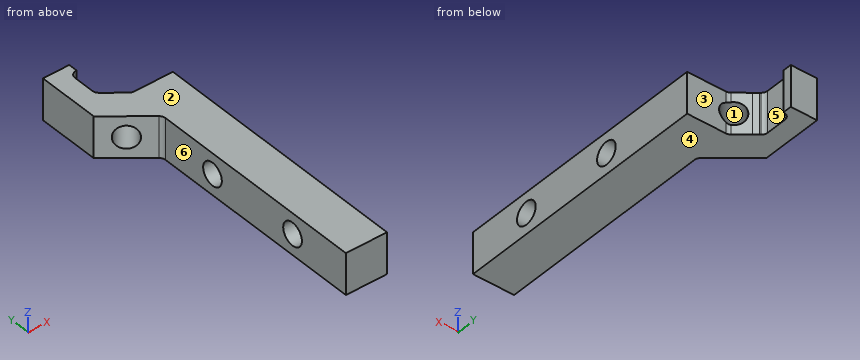
from build123d import *

# Parameters (mm, degrees)
BOSS_EXTRUDE1_DEPTH     = 12.7
CUT_EXTRUDE1_DEPTH      = 100.645019946
CUT_EXTRUDE1_DEPTH_BACK = 100.645019946
SKETCH6_R               = 3.5
SKETCH8_R               = 3.5
CUT_EXTRUDE2_DEPTH      = 315.511656717


with BuildPart() as part:
    # Sketch1 → Boss-Extrude1 (new body)
    with BuildSketch(Plane.XY):
        with BuildLine():
            Line((-312.7, 0), (-300, 0))
            Line((-300, 0), (-300, 80.249402298))
            Line((-300, 80.249402298), (-311.985474591, 80.249402298))
            ThreePointArc((-311.985474591, 80.249402298), (-312.658347569, 80.365989981), (-313.252771846, 80.702160342))
            Line((-313.252771846, 80.702160342), (-317.170141731, 83.91075489))
            Line((-317.170141731, 83.91075489), (-318.5, 85))
            Line((-318.5, 85), (-318.767297255, 85.21893478))
            ThreePointArc((-318.767297255, 85.21893478), (-319.307566667, 85.91019616), (-319.5, 86.766176735))
            Line((-319.5, 86.766176735), (-319.5, 93.25))
            ThreePointArc((-319.5, 93.25), (-318.914213562, 94.664213562), (-317.5, 95.25))
            Line((-317.5, 95.25), (-317.388555411, 95.25))
            Line((-317.388555411, 95.25), (-317.388555411, 96.25))
            Line((-317.388555411, 96.25), (-317.388555411, 98))
            Line((-317.388555411, 98), (-318.5, 98))
            Line((-318.5, 98), (-325.5, 98))
            Line((-325.5, 98), (-325.5, 85))
            Line((-325.5, 85), (-325.5, 82))
            Line((-325.5, 82), (-325.5, 79))
            Line((-325.5, 79), (-313.432702745, 69.116056102))
            ThreePointArc((-313.432702745, 69.116056102), (-312.892433333, 68.424794722), (-312.7, 67.568814146))
            Line((-312.7, 67.568814146), (-312.7, 63.3))
            Line((-312.7, 63.3), (-312.7, 60.3))
            Line((-312.7, 60.3), (-312.7, 0))
        make_face()
    extrude(amount=BOSS_EXTRUDE1_DEPTH)

    # Sketch6 → Cut-Extrude1 (cut, two sides: drawn at the far end of the back side and taken through both)
    with BuildSketch(Plane.ZY.offset(312.7).offset(-CUT_EXTRUDE1_DEPTH_BACK)):
        with Locations((6.35, 50)):
            Circle(SKETCH6_R)
        with Locations((6.35, 20)):
            Circle(SKETCH6_R)
    extrude(amount=CUT_EXTRUDE1_DEPTH + CUT_EXTRUDE1_DEPTH_BACK, mode=Mode.SUBTRACT)

    # Sketch8 → Cut-Extrude2 (cut, through all)
    with BuildSketch(Plane(origin=(-91.96558898, -112.280695929, 0), x_dir=(0.7736209776319443, -0.6336486273699289, 0), z_dir=(-0.6336486273699289, -0.7736209776319443, 0))):
        with Locations((-294.07263889, 6.35)):
            Circle(SKETCH8_R)
    extrude(amount=-CUT_EXTRUDE2_DEPTH, mode=Mode.SUBTRACT)


solid = part.part
Work out the finished part from the listing and answer in its coordinate system (mm). Face numbers are marked on the shaded views. A direction names the side the tool comes from. Give positions to 0.01 mm unless a question says otherwise; leave off trailing zeros. Write each loop counter-clockwise with the first axis right and the second up, starting at its lowest first coordinate (ties: lowest second). Pieces come first, ordered by that corner, then holes.
Q1. For a pull along Y with two mould halves and no side action, classify the marked faces 1, 2 and 3 as released by +Y, released by -Y, zero draft, split by the parting line, or undercut.
Answer:
face 1: undercut
face 2: zero draft
face 3: released by +Y
Q2. A tool of negligible diameter and unlimited length cuts with its end or side. For the marked faces 4, 5 and 6, from which of +Z, -Z, +X, -X, +Y, -Y can it reach the whole face along a straight path? Write none if from no direction.
Answer:
face 4: -Z, +X, -X, +Y, -Y
face 5: +Z, -Z, +X
face 6: +Z, -Z, -X, -Y
Q3. The part is cut by section C-C on z = 5. Give the vertices of the cut face in (x, y), and give its area (3 significant figures).
Answer:
outline: (-325.5, 79) - (-321.96, 76.1) - (-316.21, 83.13) - (-318.77, 85.22) arc R2 cw to (-319.5, 86.77) - (-319.5, 93.25) arc R2 cw to (-317.5, 95.25) - (-317.39, 95.25) - (-317.39, 98) - (-325.5, 98) - close; (-316.97, 72.01) - (-313.43, 69.12) arc R2 cw to (-312.7, 67.57) - (-312.7, 53.23) - (-300, 53.23) - (-300, 80.25) - (-310.22, 80.25) - close; (-312.7, 0) - (-300, 0) - (-300, 16.77) - (-312.7, 16.77) - close; (-312.7, 23.23) - (-300, 23.23) - (-300, 46.77) - (-312.7, 46.77) - close
area: 1,010 mm2
Q4. The part is cut by section D-D on z = 11.25. Give the vertices of the cut face in (x, y).
Answer:
outline: (-325.5, 79) - (-313.43, 69.12) arc R2 cw to (-312.7, 67.57) - (-312.7, 0) - (-300, 0) - (-300, 80.25) - (-311.99, 80.25) arc R2 cw to (-313.25, 80.7) - (-318.77, 85.22) arc R2 cw to (-319.5, 86.77) - (-319.5, 93.25) arc R2 cw to (-317.5, 95.25) - (-317.39, 95.25) - (-317.39, 98) - (-325.5, 98) - close
Q5. The part is cut by section A-A on x = -302.5. Give the vertices of the cut face in (y, z), and give its area (3 significant figures).
Answer:
outline: (0, 0) - (80.25, 0) - (80.25, 12.7) - (0, 12.7) - close; hole circle Ø7 at (20, 6.35); hole circle Ø7 at (50, 6.35)
area: 942 mm2
Q6. Straight lines are drawn through the part: L1, parallel to Y at x = -306.5, z = 6.35; L2, parallel to Z at x = -305.5, y = 20; L3, parallel to X at y = 38, z = 6. For each, find the intervals that lie inside material, in ascending order.
Answer:
L1: y = 0 to 16.5, 23.5 to 46.5, 53.5 to 80.25
L2: z = 0 to 2.85, 9.85 to 12.7
L3: x = -312.7 to -300
Q7. The part is cut by section B-B on y = 20. Give the vertices of the cut face in (x, z).
Answer:
outline: (-312.7, 0) - (-300, 0) - (-300, 2.85) - (-312.7, 2.85) - close; (-312.7, 9.85) - (-300, 9.85) - (-300, 12.7) - (-312.7, 12.7) - close
Q8. Given pin 1 (5 mm diameter, centred on y = 91.5, z = 4, fed in from +X); pin 2 (5.5 mm diameter, centred on y = 50, z = 6.35, fed in from +X) (1 decimal); pin 3 (0.8 mm diameter, centred on y = 96, z = 8, fed in from +X); pin 4 (3 mm diameter, centred on x = -305.5, z = 9, fed in from +Y), each flat-ended and moving along its own axis, determine where each tip first touches the part or whether it passes through.
Answer:
pin 1: stops at x = -319.35
pin 2: passes through
pin 3: stops at x = -317.39
pin 4: stops at y = 80.25
